Autodesk Inventor part; units mm, degrees
ref_plane "YZ Plane" through (0, 0, 0) normal (1, 0, 0) x (0, 1, 0)
ref_plane "XZ Plane" through (0, 0, 0) normal (0, 1, 0) x (-1, 0, 0)
ref_plane "XY Plane" through (0, 0, 0) normal (0, 0, 1) x (1, 0, 0)
sketch "Sketch1" plane through (0, 0, 0) normal (0, 0, 1) x (1, 0, 0)
  line L0 (0, 10) -> (10, 10)
  line L1 (10, 10) -> (10, 15)
  line L2 (10, 15) -> (12, 15)
  line L3 (12, 15) -> (12, 7.5)
  line L4 (12, 7.5) -> (15, 7.5)
  line L5 (0, 0) -> (21.5925, 0)
  line L6 (0, 10) -> (0, 3.9)
  line L7 (0, 3.9) -> (15, 3.9)
  line L8 (15, 7.5) -> (15, 3.9)
  point P0 (12, 11.25)
  dimension "d0" = 20
  dimension "d1" = 7.8
  dimension "d3" = 30
  dimension "d4" = 15
  dimension "d6" = 10
  dimension "d7" = 2
  dimension "d10" = 3
revolve "Revolution1" add sketch "Sketch1" angle 360 about axis through (0, 0, 0) along (1, 0, 0)
properties part number "SensorSkiva Plugg"
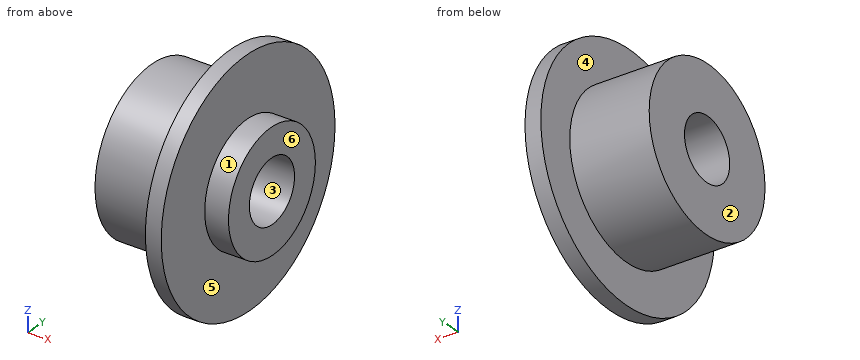
Can you work these out from the model? Positions are in its coordinate system, mm. Face numbers are marked on the shaded views. A direction names the side the tool comes from. Round coordinates to 2 decimals unless told otherwise and drop trailing zeros. Order: outer loops, then holes, each group sorted by start corner. A loop starts at its lowest first (then second) coordinate and runs counter-clockwise, first axis right, second up. Notation, with made-up numbers: (-10, 39.5) - (23, 39.5) arc R25 cw to (23, 70.5) - close; hole circle Ø4 at (3, 73). An arc over 180 degrees is marked (long way). Answer in a Markdown table with one row per item.
(1) If we mould it in two halves opening along Z, with no side actions, what happens to the marked faces 1, 2 and 3? For each: released by +Z, released by -Z, zero draft, split by the parting line, or undercut.
From the geometry:
| item | result |
|---|---|
| face 1 | split by the parting line |
| face 2 | zero draft |
| face 3 | undercut |
(2) Suppose I cut it at D-D, the plane y = 9. Please give me the cut outline in (x, z), plus the area to 3 significant figures.
From the geometry:
| item | result |
|---|---|
| outline | (0, -4.36) - (10, -4.36) - (10, -12) - (12, -12) - (12, 12) - (10, 12) - (10, 4.36) - (0, 4.36) - close |
| area | 135 mm2 |
(3) Suppose I cut it at C-C, the plane x = 11.25. Please give me the cut outline in (y, z), plus the area to 3 significant figures.
From the geometry:
| item | result |
|---|---|
| outline | circle Ø30 at (0, 0); hole circle Ø7.8 at (0, 0) |
| area | 659 mm2 |
(4) Which directions (+Z, -Z, +X, -X, +Y, -Y) give clear straight access to the entire face, cutting with the end or side of a thin tool? Please do the marked faces 4, 5 and 6.
From the geometry:
| item | result |
|---|---|
| face 4 | -X |
| face 5 | +X |
| face 6 | +Z, -Z, +X, +Y, -Y |
(5) For P1, Ø3, axis at x = 1.5, z = -0.5, coming from the +Y side; P2, Ø2, axis at x = 9.5, z = -11.5, coming from the +Y side; P3, Ø6, axis at y = -7.5, z = 9.5, coming from the +X side, each with a flat end and sliding along its axis, tell me the tip position at first contact or that it passes through.
From the geometry:
| item | result |
|---|---|
| P1 | stops at y = 10 |
| P2 | stops at y = 10.58 |
| P3 | stops at x = 12 |
(6) Please list where these lines run through material, in increasing order: L1, parallel to Z at x = 3.75, y = 0; L2, parallel to Z at x = 9, y = 2; L3, parallel to X at y = 6, z = 10. Write a range as from..to.
From the geometry:
| item | result |
|---|---|
| L1 | z = -10..-3.9, 3.9..10 |
| L2 | z = -9.8..-3.35, 3.35..9.8 |
| L3 | x = 10..12 |
(7) Suppose I cut it at A-A, the plane z = 0. Please give me the cut outline in (x, y), plus the area to 3 significant figures.
From the geometry:
| item | result |
|---|---|
| outline | (0, -10) - (10, -10) - (10, -15) - (12, -15) - (12, -7.5) - (15, -7.5) - (15, -3.9) - (0, -3.9) - close; (0, 3.9) - (15, 3.9) - (15, 7.5) - (12, 7.5) - (12, 15) - (10, 15) - (10, 10) - (0, 10) - close |
| area | 188 mm2 |
